from build123d import *

# Parameters (mm, degrees)
SKETCH1_R           = 5.5
SKETCH1_R_2         = 3.5
BOSS_EXTRUDE1_DEPTH = 40
SKETCH2_W           = 5
SKETCH2_H           = 10
CUT_EXTRUDE1_DEPTH  = 20
SKETCH3_R           = 0.75
CUT_EXTRUDE2_DEPTH  = 10


with BuildPart() as part:
    # Sketch1 → Boss-Extrude1 (new body)
    with BuildSketch(Plane(origin=(0, 0, 0), x_dir=(1, 0, 0), z_dir=(0, 1, 0))):
        with Locations(Location((0, 0, 0), (0, 0, 270))):
            Circle(SKETCH1_R)
        with Locations(Location((0, 0, 0), (0, 0, 270))):
            Circle(SKETCH1_R_2, mode=Mode.SUBTRACT)
    extrude(amount=BOSS_EXTRUDE1_DEPTH)

    # Sketch2 → Cut-Extrude1 (cut, symmetric)
    with BuildSketch(Plane.XY):
        with Locations((0, 35)):
            Rectangle(SKETCH2_W, SKETCH2_H)
        with Locations((0, 45)):
            Rectangle(SKETCH2_W, SKETCH2_H)
    extrude(amount=CUT_EXTRUDE1_DEPTH, both=True, mode=Mode.SUBTRACT)

    # Sketch3 → Cut-Extrude2 (cut, symmetric)
    with BuildSketch(Plane(origin=(0, 0, 0), x_dir=(0, 0, -1), z_dir=(1, 0, 0))):
        with Locations(Location((0, 36, 0), (0, 0, 180))):
            Circle(SKETCH3_R)
    extrude(amount=CUT_EXTRUDE2_DEPTH, both=True, mode=Mode.SUBTRACT)


solid = part.part
Model file for the job. Use its own axes, mm. A direction names the side the tool comes from. Give positions to 0.01 mm unless a question says otherwise; leave off trailing zeros. Order: outer loops, then holes, each group sorted by start corner. A loop starts at its lowest first (then second) coordinate and runs counter-clockwise, first axis right, second up. Notation, with made-up numbers: (-20, 21) - (2, 21) arc R10 cw to (2, 33) - close; hole circle Ø1 at (85.25, 69). An arc over 180 degrees is marked (long way). One line per item, written item: value.
Item 1: Two-plate mould, pull along X, no slides. Class faces 1 (the flat face through (0, 0, 4)), 2 (the flat face through (0, 30, -4)), 3 (the cylindrical face through (0.242, 19.72, -5.495)): released by +X, released by -X, zero draft, split by the parting line, or undercut.
Response values:
face 1: zero draft
face 2: undercut
face 3: split by the parting line
Item 2: Slice it at C-C (z = -2). List the corners of the cut face in (x, y).
Response values:
outline: (-5.12, 0) - (-2.87, 0) - (-2.87, 40) - (-5.12, 40) - close; (2.87, 0) - (5.12, 0) - (5.12, 40) - (2.87, 40) - close
Item 3: Slice it at B-B (x = 0). List the corners of the cut face in (y, z).
Response values:
outline: (0, -5.5) - (30, -5.5) - (30, -3.5) - (0, -3.5) - close; (0, 3.5) - (30, 3.5) - (30, 5.5) - (0, 5.5) - close
Item 4: Pin check, flat tips, straight feed: pin 1 Ø2.5 at (x, z) = (-0.5, 4.5) entering from +Y; pin 2 Ø6 at (x, y) = (-2.5, 28.5) entering from -Z; pin 3 Ø1.2 at (y, z) = (33, -3.5) entering from -X; pin 4 Ø0.7 at (y, z) = (36, -4) entering from +X. Stop position of each tip, or through.
Response values:
pin 1: y = 30
pin 2: z = -5.5
pin 3: x = -4.67
pin 4: x = 4.11
Item 5: Tool access for faces 4 (the flat face through (-2.5, 35, -4)), 5 (the cylindrical face through (4.474, 35.368, 0.403)): list every direction of +Z, -Z, +X, -X, +Y, -Y with a clear straight run to the whole face (end or side of a thin tool).
Response values:
face 4: +Z, -Z, +Y
face 5: +X, -X
Item 6: Slice it at A-A (z = 0). List the corners of the cut face in (x, y), then the cut area to 3 significant figures.
Response values:
outline: (-5.5, 0) - (-3.5, 0) - (-3.5, 35.25) - (-5.5, 35.25) - close; (-5.5, 36.75) - (-3.5, 36.75) - (-3.5, 40) - (-5.5, 40) - close; (3.5, 0) - (5.5, 0) - (5.5, 35.25) - (3.5, 35.25) - close; (3.5, 36.75) - (5.5, 36.75) - (5.5, 40) - (3.5, 40) - close
area: 154 mm2
Item 7: Wall check: line 1 (X direction, y = 26.5, z = 0); line 2 (X direction, y = 24.5, z = -2.5); line 3 (Y direction, x = -1.5, z = -3.5). Give the ranges that are in metal, low to high.
Response values:
line 1: -5.5 to -3.5, 3.5 to 5.5
line 2: -4.9 to -2.45, 2.45 to 4.9
line 3: 0 to 30
Item 8: Slice it at D-D (y = 36). List the corners of the cut face in (x, z), then the cut area to 3 significant figures.
Response values:
outline: (-5.45, -0.75) arc R5.5 ccw to (-2.5, -4.9) - (-2.5, -2.45) arc R3.5 cw to (-3.42, -0.75) - close; (-5.45, 0.75) - (-3.42, 0.75) arc R3.5 cw to (-2.5, 2.45) - (-2.5, 4.9) arc R5.5 ccw to start; (2.5, -4.9) arc R5.5 ccw to (5.45, -0.75) - (3.42, -0.75) arc R3.5 cw to (2.5, -2.45) - close; (2.5, 2.45) arc R3.5 cw to (3.42, 0.75) - (5.45, 0.75) arc R5.5 ccw to (2.5, 4.9) - close
area: 29.2 mm2
